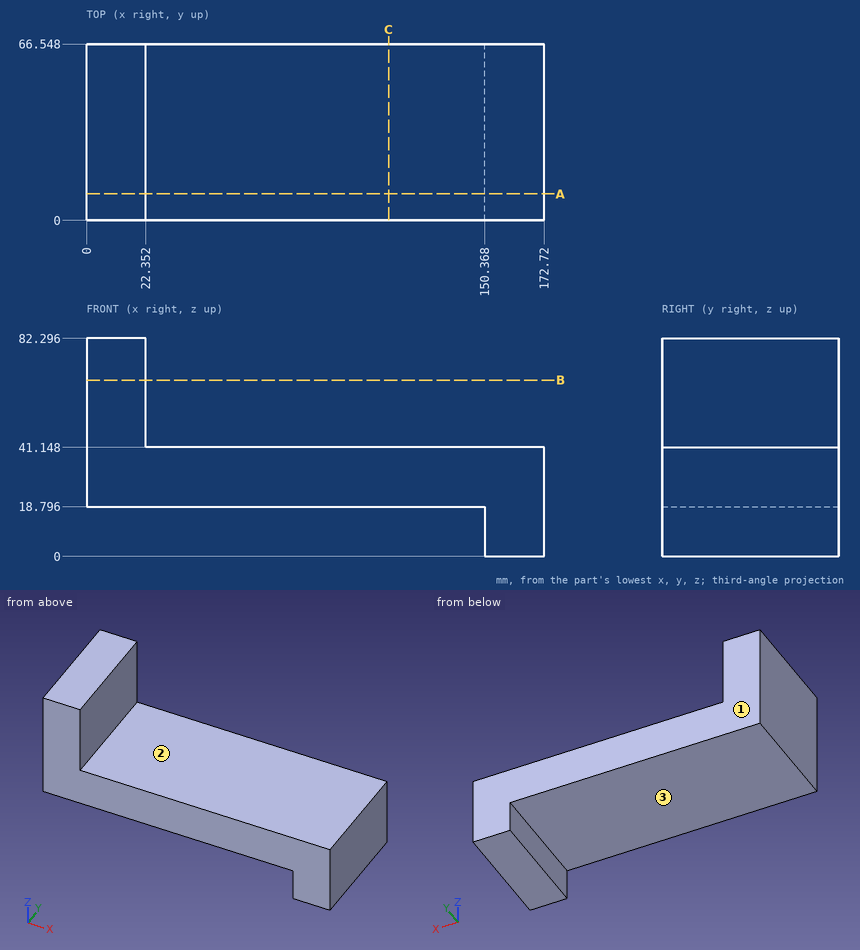
Print and shaded views of the part. All mm, measured from the part's lowest x, y and z. A direction names the side the tool comes from. Give positions to 0.01 mm unless a question says otherwise; leave off trailing zeros. Loops run counter-clockwise (first coordinate to the right, second up) from the corner with the lowest first, then second, coordinate; pieces in that order, holes last. Notation, with made-up numbers: (33, 23.25) - (42, 23.25) arc R22 ccw to (42, 56.25) - close; hole circle Ø10 at (-24, -12). An arc over 180 degrees is marked (long way). Use a Markdown table: item, result.
(1) Drop flat-ended pins along their axis: pin 1 Ø10 at (y, z) = (28.5, 44.5) entering from +X; pin 2 Ø5 at (x, y) = (62, 45.5) entering from -Z; pin 3 Ø9.5 at (y, z) = (34.5, 11) entering from -X. Give the stop position or say it passes through.
Taken from the geometry:
| item | result |
|---|---|
| pin 1 | x = 172.72 |
| pin 2 | z = 18.8 |
| pin 3 | x = 150.37 |
(2) Band-saw the part on C-C (x = 114). Give the cut face in (y, z).
Taken from the geometry:
| item | result |
|---|---|
| outline | (0, 18.8) - (66.55, 18.8) - (66.55, 41.15) - (0, 41.15) - close |
(3) Band-saw the part on B-B (z = 66.5). Give the cut face in (x, y), and give its area (3 significant figures).
Taken from the geometry:
| item | result |
|---|---|
| outline | (0, 0) - (22.35, 0) - (22.35, 66.55) - (0, 66.55) - close |
| area | 1,490 mm2 |
(4) Wall check: line 1 along X through (y, z) = (16.5, 9); line 2 along X through (y, z) = (17.5, 73.5); line 3 along Z through (x, y) = (56.5, 23). Give the ranges that are in metal, low to high.
Taken from the geometry:
| item | result |
|---|---|
| line 1 | 150.37 to 172.72 |
| line 2 | 0 to 22.35 |
| line 3 | 18.8 to 41.15 |
(5) Band-saw the part on A-A (y = 10). Give the cut face in (x, z), and give its area (3 significant figures).
Taken from the geometry:
| item | result |
|---|---|
| outline | (0, 18.8) - (150.37, 18.8) - (150.37, 0) - (172.72, 0) - (172.72, 41.15) - (22.35, 41.15) - (22.35, 82.3) - (0, 82.3) - close |
| area | 5,200 mm2 |
(6) Which spindle directions (+Z, -Z, +X, -X, +Y, -Y) get a long thin tool onto all of the face, cutting with end or side? Do the marked faces 1, 2 and 3. Say none if no direction does.
Taken from the geometry:
| item | result |
|---|---|
| face 1 | +Z, -Z, +X, -X, +Y |
| face 2 | +Z, +X, +Y, -Y |
| face 3 | -Z, -X, +Y, -Y |
